Autodesk Inventor part; units mm, degrees
ref_plane "YZ Plane" through (0, 0, 0) normal (1, 0, 0) x (0, 1, 0)
ref_plane "XZ Plane" through (0, 0, 0) normal (0, 1, 0) x (-1, 0, 0)
ref_plane "XY Plane" through (0, 0, 0) normal (0, 0, 1) x (1, 0, 0)
sketch "Sketch1" plane through (0, 0, 0) normal (0, 1, 0) x (-1, 0, 0)
  line L0 (21.7482, 13.5362) -> (21.7482, 19.7862)
  line L1 (21.7482, 19.7862) -> (-5.2518, 19.7862)
  line L2 (-5.2518, 19.7862) -> (-5.2518, -15.7138)
  line L3 (-5.2518, -15.7138) -> (0.7482, -15.7138)
  line L4 (0.7482, -15.7138) -> (0.7482, -19.9638)
  line L5 (0.7482, -19.9638) -> (2.7482, -19.9638)
  line L6 (4.7482, -13.7138) -> (-3.2518, -13.7138)
  line L7 (-3.2518, -13.7138) -> (-3.2518, 17.7862)
  line L8 (-3.2518, 17.7862) -> (19.7482, 17.7862)
  line L9 (19.7482, 17.7862) -> (19.7482, 13.5362)
  line L10 (19.7482, 13.5362) -> (21.7482, 13.5362)
  line L11 (4.7482, -13.7138) -> (4.7482, -15.7138)
  line L12 (4.7482, -15.7138) -> (2.7482, -15.7138)
  line L13 (2.7482, -15.7138) -> (2.7482, -19.9638)
  point P0 (0, 0)
  dimension "d1" = 4.25
  dimension "d2" = 2
  dimension "d3" = 2
  dimension "d4" = 2
  dimension "d5" = 2
  dimension "d6" = 2
  dimension "d7" = 23
  dimension "d8" = 2
  dimension "d9" = 4.25
  dimension "d10" = 2
  dimension "d21" = 31.5
  dimension "d22" = 8
extrude "Extrusion1" add sketch "Sketch1" along normal blind 12
sketch "Sketch2" plane through (-21.7482, 0, 13.5362) normal (-1, 0, 0) x (0, 0, 1)
  circle A0 centre (2.5, 6) radius 1
  line L0 (6.25, 0) -> (6.25, 12)
  line L1 (0, 0) -> (0, 12)
  point P0 (-13.5362, 0)
  point P1 (6.25, 6)
  dimension "d13" = 1.5
  dimension "d14" = 2
extrude "Extrusion2" cut sketch "Sketch2" against normal up to surface (2 mm away)
sketch "Sketch3" plane through (-2.7482, 0, -19.9638) normal (-1, 0, 0) x (0, 0, 1)
  circle A0 centre (2.5, 6) radius 1
  line L0 (0, 0) -> (0, 12)
  point P0 (19.9638, 0)
  point P1 (0, 6)
  dimension "d17" = 1.5
  dimension "d18" = 2
extrude "Extrusion3" cut sketch "Sketch3" against normal up to surface (2 mm away)
chamfer "Chamfer1" distance 1 angle 45 13 edges at (5.2518, 0, 2.0362) (5.2518, 12, 2.0362) (-8.2482, 12, 19.7862) (-8.2482, 0, 19.7862) (-21.7482, 0, 16.6612) (-21.7482, 12, 16.6612) (-21.7482, 6, 19.7862) (5.2518, 6, -15.7138) (2.2518, 12, -15.7138) (2.2518, 0, -15.7138) (-0.7482, 12, -17.8388) (-0.7482, 0, -17.8388) (5.2518, 6, 19.7862)
sketch "Sketch4" plane through (5.2518, 1, -14.7138) normal (1, 0, 0) x (0, 0, -1)
  circle A0 centre (2.75, 5) radius 2.5
  circle A1 centre (2.75, 5) radius 1
  point P0 (-14.7138, -1)
  dimension "d26" = 5
extrude "Extrusion4" cut sketch "Sketch4" against normal up to surface (6 mm away) contours A0 | A1
equation "\"d1\" = -0.5 * servo_A + 0.5 * servo_D"
equation "\"d7\" = servo_E + servo_F"
equation "\"d8\" = servo_F"
equation "\"d9\" = -0.5 * servo_A + 0.5 * servo_D"
equation "\"d21\" = servo_D"
equation "\"d11\" = servo_B"
equation "\"d13\" = servo_L"
equation "\"d14\" = servo_H"
equation "\"d15\" = servo_B"
equation "\"d17\" = servo_L"
equation "\"d18\" = servo_H"
equation "\"d19\" = servo_B"
properties part number "FEMUR2_B"
Verification items for the finished model (mm, model axes). A direction names the side the tool comes from. Coordinates: 2 decimals unless noted, no trailing zeros. Order: outer loops, then holes, each group sorted by start corner. A loop starts at its lowest first (then second) coordinate and runs counter-clockwise, first axis right, second up. Notation, with made-up numbers: (75.25, -6) -> (120.25, -6) arc R17 cw to (120.25, 0) -> close; hole circle Ø4 at (-34, -9.5). An arc over 180 degrees is marked (long way). Use CSV: the item, a comma, the result in double quotes. Start each with the question number.
Q1. Tool access check on faces 1 (the flat face through (-4, 6, -15.714)), 2 (the cylindrical face through (2.168, 6.028, -14.964)), 3 (the flat face through (-1, 6, -13.714)), 4 (the flat face through (-19.748, 5.9, 14.7)), 5 (the flat face through (-8, 6, 17.786)). Record the directions out of +Z, -Z, +X, -X, +Y, -Y that give a thin tool (end or side, any length) a straight path to the whole face; none if there is none.
Q2. Depth check by flat-ended pin: P1, Ø3, axis at y = 6.5, z = 2.5, coming from the -X side; P2, Ø0.6, axis at x = -21, y = 8, coming from the -Z side; P3, Ø2, axis at y = 6.5, z = -15, coming from the -X side. Enter the tip coordinate at first touch or a pass-through.
Q3. Section check B-B, the plane y = 6. Record the cut outline in (x, z), and give its area (3 significant figures).
Q4. Thickness scan on line 1 along Z through (x, y) = (-1.5, 8.5); line 2 along X through (y, z) = (6.5, -14.5); line 3 along X through (y, z) = (2.25, -9.5). Record the ranges inside material, lowest first.
Q5. Section check D-D, the plane z = -17. Record the cut outline in (x, y), and give its area (3 significant figures).
Q6. Draft check along Z on faces 6 (the flat face through (4.87, 4.819, -15.096)), 7 (the flat face through (3.252, 6, 2)), 8 (the flat face through (-21.13, 0.684, 19.088)), 9 (the flat face through (-0.748, 6, -19)). Enter one of: +Z half, -Z half, draft (parallel to the pull), parting line (faces both ways), or undercut.
Q7. Section check C-C, the plane y = 8.25. Record the cut outline in (x, z), and give its area (4 significant figures).
Q8. Section check A-A, the plane x = 2.75. Record the cut outline in (y, z), and give its area (3 significant figures).
Returned:
1,face 1,"-Z, -X, +Y, -Y"
1,face 2,"-Z, +X"
1,face 3,"-X, +Y, -Y"
1,face 4,"-Z, +Y, -Y"
1,face 5,"+Y, -Y"
2,P1,"stops at x = 3.25"
2,P2,"stops at z = 13.54"
2,P3,"stops at x = -4.75"
3,outline,"(-21.75, 13.54) -> (-19.75, 13.54) -> (-19.75, 15.04) -> (-21.75, 15.04) -> close; (-21.75, 17.04) -> (-19.75, 17.04) -> (-19.75, 17.79) -> (3.25, 17.79) -> (3.25, -13.71) -> (-4.75, -13.71) -> (-4.75, -15.71) -> (-2.75, -15.71) -> (-2.75, -16.46) -> (-0.75, -16.46) -> (-0.75, -14.96) -> (5, -14.96) -> (5.25, -14.71) -> (5.25, 18.79) -> (4.25, 19.79) -> (-20.75, 19.79) -> (-21.75, 18.79) -> close; (-2.75, -19.96) -> (-0.75, -19.96) -> (-0.75, -18.46) -> (-2.75, -18.46) -> close"
3,area,"140 mm^2"
4,line 1,"z = -19.96 to -13.71, 17.79 to 19.79"
4,line 2,"x = -4.75 to 5.25"
4,line 3,"x = 3.25 to 5.25"
5,outline,"(-2.75, 0) -> (-1.75, 0) -> (-0.75, 1) -> (-0.75, 5.11) -> (-2.75, 5.11) -> close; (-2.75, 6.89) -> (-0.75, 6.89) -> (-0.75, 11) -> (-1.75, 12) -> (-2.75, 12) -> close"
5,area,"19.5 mm^2"
6,face 6,"-Z half"
6,face 7,"undercut"
6,face 8,"+Z half"
6,face 9,"draft"
7,outline,"(-21.75, 13.54) -> (-19.75, 13.54) -> (-19.75, 17.79) -> (3.25, 17.79) -> (3.25, -13.71) -> (-4.75, -13.71) -> (-4.75, -15.71) -> (-2.75, -15.71) -> (-2.75, -19.96) -> (-0.75, -19.96) -> (-0.75, -15.71) -> (4.25, -15.71) -> (5.25, -14.71) -> (5.25, 18.79) -> (4.25, 19.79) -> (-20.75, 19.79) -> (-21.75, 18.79) -> close"
7,area,"152.5 mm^2"
8,outline,"(0, -14.71) -> (1, -15.71) -> (4.21, -15.71) arc R2.5 cw to (7.79, -15.71) -> (11, -15.71) -> (12, -14.71) -> (12, -13.71) -> (0, -13.71) -> close; (0, 17.79) -> (12, 17.79) -> (12, 18.79) -> (11, 19.79) -> (1, 19.79) -> (0, 18.79) -> close"
8,area,"44.2 mm^2"
